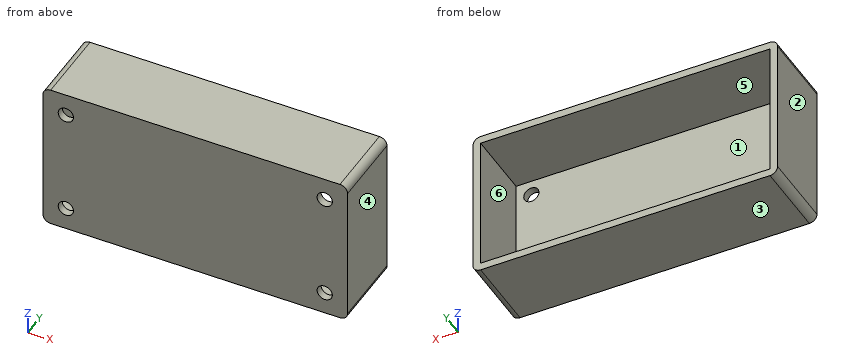
```python
from build123d import *

# Parameters (mm, degrees)
SKETCH1_W           = 200
SKETCH1_H           = 100
BOSS_EXTRUDE1_DEPTH = 50
SHELL1_T            = -5
FILLET1_R           = 5
SKETCH5_R           = 5
CUT_EXTRUDE1_DEPTH  = 6


with BuildPart() as part:
    # Sketch1 → Boss-Extrude1 (new body)
    with BuildSketch(Plane(origin=(0, 0, 0), x_dir=(1, 0, 0), z_dir=(0, 1, 0))):
        Rectangle(SKETCH1_W, SKETCH1_H)
    extrude(amount=BOSS_EXTRUDE1_DEPTH)

    # Shell1
    shell1_openings = [part.faces().sort_by_distance(p)[0] for p in [
        (0, 50, 0),
    ]]
    offset(amount=SHELL1_T, openings=shell1_openings, kind=Kind.INTERSECTION)

    # Fillet1
    fillet1_edges = [part.edges().sort_by_distance(p)[0] for p in [
        (-100, 25, -50),
        (100, 25, -50),
        (100, 25, 50),
        (-100, 25, 50),
    ]]
    fillet(fillet1_edges, radius=FILLET1_R)

    # Sketch5 → Cut-Extrude1 (cut, through all)
    with BuildSketch(Plane(origin=(0, 5, 0), x_dir=(1, 0, 0), z_dir=(0, 1, 0))):
        with Locations((-85, 35)):
            Circle(SKETCH5_R)
        with Locations((85, 35)):
            Circle(SKETCH5_R)
        with Locations((85, -35)):
            Circle(SKETCH5_R)
        with Locations((-85, -35)):
            Circle(SKETCH5_R)
    extrude(amount=-CUT_EXTRUDE1_DEPTH, mode=Mode.SUBTRACT)


solid = part.part
```
Here's how the part is built. I have some questions about the finished solid (model axes, mm). Face numbers are marked on the shaded views. A direction names the side the tool comes from. Round coordinates to 2 decimals unless told otherwise and drop trailing zeros. Write each loop counter-clockwise with the first axis right and the second up, starting at its lowest first coordinate (ties: lowest second). Pieces come first, ordered by that corner, then holes.
Q1. If we section it at C-C on x = 85: Write out the boundary of the cut face in (y, z).
Q2. Will this pin go through, and if not, where does the flat tip stop? P1, Ø8, axis at x = 36.5, z = -20.5, coming from the +Y side.
Q3. If we section it at A-A on y = 38.5: Write out the boundary of the cut face in (x, z), plus the area to 3 significant figures.
Q4. Which directions (+Z, -Z, +X, -X, +Y, -Y) give clear straight access to the entire face, cutting with the end or side of a thin tool? Please do the marked faces 1 and 2.
Q5. Please list where these lines run through material, in increasing order: probe 1 along Z at (x, y) = (85, 2.65); probe 2 along X at (y, z) = (1, 35); probe 3 along Z at (x, y) = (-52.5, 35).
Q6. If we mould it in two halves opening along X, with no side actions, what happens to the marked faces 3, 4, 5 and 6? For each: +X half, -X half, draft (parallel to the pull), parting line (faces both ways), or undercut.
Q7. If we section it at B-B on z = -35: Write out the boundary of the cut face in (x, y).
Q8. If we section it at D-D on z = -18.5: Write out the boundary of the cut face in (x, y).
Answer below:
1. outline: (0, -50) - (50, -50) - (50, -45) - (5, -45) - (5, -40) - (0, -40) - close; (0, -30) - (5, -30) - (5, 30) - (0, 30) - close; (0, 40) - (5, 40) - (5, 45) - (50, 45) - (50, 50) - (0, 50) - close
2. P1: stops at y = 5
3. outline: (-100, -45) arc R5 ccw to (-95, -50) - (95, -50) arc R5 ccw to (100, -45) - (100, 45) arc R5 ccw to (95, 50) - (-95, 50) arc R5 ccw to (-100, 45) - close; hole (-95, -45) - (95, -45) - (95, 45) - (-95, 45) - close
3. area: 2,880 mm2
4. face 1: +Y
4. face 2: +Z, -Z, -X, +Y, -Y
5. probe 1: z = -50 to -40, -30 to 30, 40 to 50
5. probe 2: x = -100 to -90, -80 to 80, 90 to 100
5. probe 3: z = -50 to -45, 45 to 50
6. face 3: draft
6. face 4: +X half
6. face 5: undercut
6. face 6: undercut
7. outline: (-100, 0) - (-90, 0) - (-90, 5) - (-95, 5) - (-95, 50) - (-100, 50) - close; (-80, 0) - (80, 0) - (80, 5) - (-80, 5) - close; (90, 0) - (100, 0) - (100, 50) - (95, 50) - (95, 5) - (90, 5) - close
8. outline: (-100, 0) - (100, 0) - (100, 50) - (95, 50) - (95, 5) - (-95, 5) - (-95, 50) - (-100, 50) - close
